Job drawing, mm, ordinate dimensions from the low corner. One solid piece. Coordinates: 2 decimals unless noted, no trailing zeros. Write each loop counter-clockwise with the first axis right and the second up, starting at its lowest first coordinate (ties: lowest second). Pieces come first, ordered by that corner, then holes. Notation, with made-up numbers: (4.25, 29) - (35.25, 29) arc R26 cw to (35.25, 67) - close; hole circle Ø5 at (-6.5, 1.25). An arc over 180 degrees is marked (long way). Use one line per item in the form item = value. Start each with the question number.
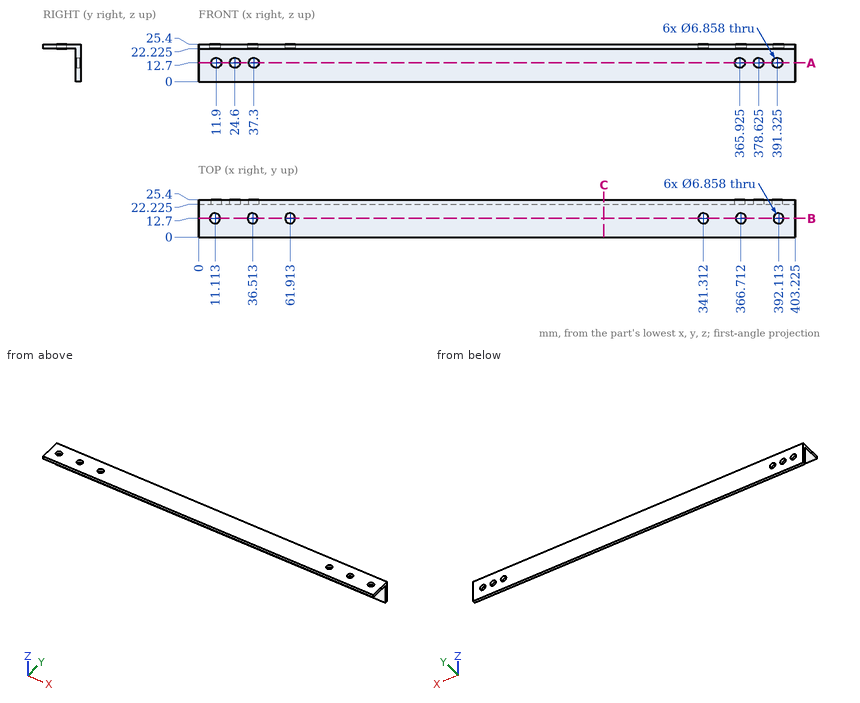
Q1. Slice it at C-C (x = 274). List the corners of the cut face in (y, z) (1 decimal), plus the area to 3 significant figures.
Q2. Pin check, flat tips, straight feed: P1, Ø11, axis at x = 378.63, z = 12.7, coming from the -Y side (1 decimal); P2, Ø8, axis at x = 75.5, y = 11, coming from the -Z side (1 decimal). Stop position of each tip, or through.
Q3. Drill centre line: probe 1 along Y at (x, z) = (186.5, 6) (1 decimal). Where is it in solid material? Low to high.
Q4. Slice it at B-B (y = 12.7). List the corners of the cut face in (x, z) (1 decimal), plus the area to 3 significant figures.
Q5. Slice it at A-A (z = 12.7). List the corners of the cut face in (x, y) (1 decimal), plus the area to 3 significant figures.
Solution:
q1.outline = (0, 22.2) - (22.2, 22.2) - (22.2, 0) - (25.4, 0) - (25.4, 25.4) - (0, 25.4) - close
q1.area = 151 mm2
q2.P1 = 22.2
q2.P2 = 22.2
q3.probe_1 = 22.2 to 25.4
q4.outline = (0, 22.2) - (7.7, 22.2) - (7.7, 25.4) - (0, 25.4) - close; (14.5, 22.2) - (33.1, 22.2) - (33.1, 25.4) - (14.5, 25.4) - close; (39.9, 22.2) - (58.5, 22.2) - (58.5, 25.4) - (39.9, 25.4) - close; (65.3, 22.2) - (337.9, 22.2) - (337.9, 25.4) - (65.3, 25.4) - close; (344.7, 22.2) - (363.3, 22.2) - (363.3, 25.4) - (344.7, 25.4) - close; (370.1, 22.2) - (388.7, 22.2) - (388.7, 25.4) - (370.1, 25.4) - close; (395.5, 22.2) - (403.2, 22.2) - (403.2, 25.4) - (395.5, 25.4) - close
q4.area = 1,150 mm2
q5.outline = (0, 22.2) - (8.5, 22.2) - (8.5, 25.4) - (0, 25.4) - close; (15.3, 22.2) - (21.2, 22.2) - (21.2, 25.4) - (15.3, 25.4) - close; (28, 22.2) - (33.9, 22.2) - (33.9, 25.4) - (28, 25.4) - close; (40.7, 22.2) - (362.5, 22.2) - (362.5, 25.4) - (40.7, 25.4) - close; (369.4, 22.2) - (375.2, 22.2) - (375.2, 25.4) - (369.4, 25.4) - close; (382.1, 22.2) - (387.9, 22.2) - (387.9, 25.4) - (382.1, 25.4) - close; (394.8, 22.2) - (403.2, 22.2) - (403.2, 25.4) - (394.8, 25.4) - close
q5.area = 1,150 mm2
